from build123d import *

# Parameters (mm, degrees)
ENL_V_START             = 20
ESQUISSE2_W             = 45.995149175
ESQUISSE2_H             = 13
ENL_V_MAT_EXTRU_1_DEPTH = 13


with BuildPart() as part:
    # Esquisse1 → Révolution1 (revolve)
    with BuildSketch(Plane.XY, mode=Mode.PRIVATE) as r_volution1_sk:
        Polygon((-44.003614869, 0), (87.477059288, 0), (87.477059288, 37.843146067), (45.995149175, 37.843146067), (45.995149175, 18.921573034), (0, 18.921573034), (0, 37.843146067), (-44.003614869, 37.843146067), align=None)
    revolve(r_volution1_sk.sketch.rotate(Axis((-44.003614869, 0, 0), (1, 0, 0)), 90), axis=Axis((-44.003614869, 0, 0), (1, 0, 0)))

    # Esquisse2 → Enlèv. mat.-Extru.1 (cut)
    with BuildSketch(Plane(origin=(0, 0, 0), x_dir=(1, 0, 0), z_dir=(0, 1, 0)).offset(ENL_V_START)):
        with Locations((22.997574588, 0)):
            Rectangle(ESQUISSE2_W, ESQUISSE2_H)
    extrude(amount=-ENL_V_MAT_EXTRU_1_DEPTH, mode=Mode.SUBTRACT)


solid = part.part
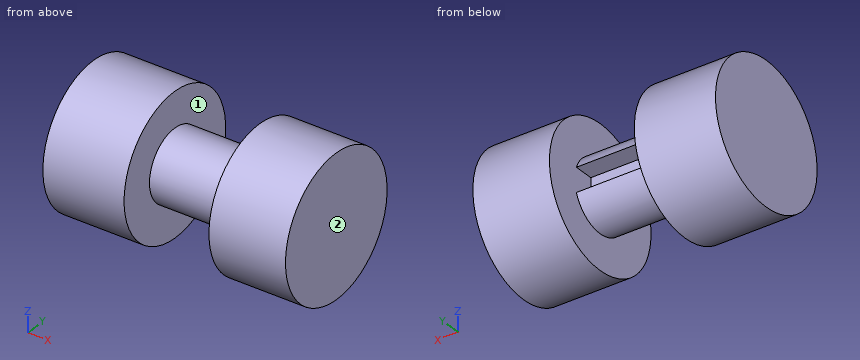
Geometry: final body of the model. Coordinates: model frame, mm. Face numbers are marked on the shaded views. A direction names the side the tool comes from. Round coordinates to 2 decimals unless told otherwise and drop trailing zeros. Write each loop counter-clockwise with the first axis right and the second up, starting at its lowest first coordinate (ties: lowest second). Pieces come first, ordered by that corner, then holes. Notation, with made-up numbers: M -8.5,-40 L 30.5,-40 A33 ccw 30.5,-9 Z; hole C 6,37.5 d1. An arc over 180 degrees is marked long. Write item = value, one per line.
Item 1: Section query D-D on y = 0. Return loops of the section in (x, z), then the cut area to 3 significant figures.
Findings:
outline = M -44,-37.84 L 0,-37.84 L 0,-18.92 L 46,-18.92 L 46,-37.84 L 87.48,-37.84 L 87.48,37.84 L 46,37.84 L 46,18.92 L 0,18.92 L 0,37.84 L -44,37.84 Z
area = 8,210 mm^2
Item 2: Pin query (flat end, axial travel): P1, Ø1.5, axis at x = 41.5, y = 20, coming from the -Z side; P2, Ø12, axis at x = 23.5, y = 15, coming from the -Z side; P3, Ø3, axis at x = 23.5, y = 10.5, coming from the +Z side; P4, Ø5, axis at x = 37, z = 13, coming from the +Y side. Return the tip coordinate at first contact, or that it passes through.
Findings:
P1 = through
P2 = -16.64
P3 = 16.64
P4 = 15.74
Item 3: Section query A-A on y = -27.5. Return loops of the section in (x, z).
Findings:
outline = M -44,-26 L 0,-26 L 0,26 L -44,26 Z; M 46,-26 L 87.48,-26 L 87.48,26 L 46,26 Z
Item 4: Section query C-C on z = 0. Return loops of the section in (x, y), then the cut area to 3 significant figures.
Findings:
outline = M -44,-37.84 L 0,-37.84 L 0,-18.92 L 46,-18.92 L 46,-37.84 L 87.48,-37.84 L 87.48,37.84 L 46,37.84 L 46,7 L 0,7 L 0,37.84 L -44,37.84 Z
area = 7,660 mm^2
Item 5: Material intervals for line 1 along X through (y, z) = (-4, -29); line 2 along Z through (x, y) = (-7, -8.5); line 3 along Y through (x, z) = (81, 22.5), sorted ascending. Write a range as [from, to].
Findings:
line_1 = [-44, 0], [46, 87.48]
line_2 = [-36.88, 36.88]
line_3 = [-30.43, 30.43]
Item 6: Access query for the marked faces 1 and 2. Directions: +Z, -Z, +X, -X, +Y, -Y. A direction counts if a zero-diameter tool reaches every point of the face in a straight line with its end or side. Return the directions, or none.
Findings:
face_1 = none
face_2 = +Z, -Z, +X, +Y, -Y
Item 7: Section query B-B on z = -28.5. Return loops of the section in (x, y).
Findings:
outline = M -44,-24.9 L 0,-24.9 L 0,24.9 L -44,24.9 Z; M 46,-24.9 L 87.48,-24.9 L 87.48,24.9 L 46,24.9 Z
